```python
from build123d import *

# Parameters (mm, degrees)
F1_DEPTH = 16
F2_R     = 7
F3_T     = -3
F5_DEPTH = 3.1
F6_R     = 0.4


with BuildPart() as f1:
    # F0 (on Top) → F1 (new body)
    with BuildSketch(Plane.XY):
        with BuildLine():
            Line((-44, -34.5), (44, -34.5))
            ThreePointArc((44, -34.5), (48.9497474683, -32.4497474683), (51, -27.5))
            Line((51, -27.5), (51, 27.5))
            ThreePointArc((51, 27.5), (48.9497474683, 32.4497474683), (44, 34.5))
            Line((44, 34.5), (-44, 34.5))
            ThreePointArc((-44, 34.5), (-48.9497474683, 32.4497474683), (-51, 27.5))
            Line((-51, 27.5), (-51, -27.5))
            ThreePointArc((-51, -27.5), (-48.9497474683, -32.4497474683), (-44, -34.5))
        make_face()
    extrude(amount=F1_DEPTH)

    # F2
    f2_edges = [f1.edges().sort_by_distance(p)[0] for p in [
        (0, -34.5, 0),
    ]]
    fillet(f2_edges, radius=F2_R)

    # F3
    f3_openings = [f1.faces().sort_by_distance(p)[0] for p in [
        (0, 0, 16),
    ]]
    offset(amount=F3_T, openings=f3_openings)

    # F4 (on face) → F5 (cut)
    with BuildSketch(Plane.XY.offset(16)):
        with BuildLine():
            Line((49.6, -27.5), (49.6, 27.5))
            ThreePointArc((49.6, 27.5), (47.9597979746, 31.4597979746), (44, 33.1))
            Line((44, 33.1), (-44, 33.1))
            ThreePointArc((-44, 33.1), (-47.9597979746, 31.4597979746), (-49.6, 27.5))
            Line((-49.6, 27.5), (-49.6, -27.5))
            ThreePointArc((-49.6, -27.5), (-47.9597979746, -31.4597979746), (-44, -33.1))
            Line((-44, -33.1), (44, -33.1))
            ThreePointArc((44, -33.1), (47.9597979746, -31.4597979746), (49.6, -27.5))
        make_face()
        with BuildLine():
            Line((-44, 31.5), (44, 31.5))
            ThreePointArc((44, 31.5), (46.8284271247, 30.3284271247), (48, 27.5))
            Line((48, 27.5), (48, -27.5))
            ThreePointArc((48, -27.5), (46.8284271247, -30.3284271247), (44, -31.5))
            Line((44, -31.5), (-44, -31.5))
            ThreePointArc((-44, -31.5), (-46.8284271247, -30.3284271247), (-48, -27.5))
            Line((-48, -27.5), (-48, 27.5))
            ThreePointArc((-48, 27.5), (-46.8284271247, 30.3284271247), (-44, 31.5))
        make_face(mode=Mode.SUBTRACT)
    extrude(amount=-F5_DEPTH, mode=Mode.SUBTRACT)

    # F6
    f6_edges = [f1.edges().sort_by_distance(p)[0] for p in [
        (0, 33.1, 12.9),
        (0, -33.1, 16),
    ]]
    fillet(f6_edges, radius=F6_R)


solid = f1.part
```
Can you work these out from the model? Positions are in its coordinate system, mm. A direction names the side the tool comes from. Give positions to 0.01 mm unless a question says otherwise; leave off trailing zeros. Write each loop counter-clockwise with the first axis right and the second up, starting at its lowest first coordinate (ties: lowest second). Pieces come first, ordered by that corner, then holes. Notation, with made-up numbers: (62, 82.5) -> (107, 82.5) arc R23 ccw to (107, 97.5) -> close; hole circle Ø8 at (-29, 40). An arc over 180 degrees is marked (long way). One line per item, written item: value.
Q1. We'd pull the mould along X, two halves only. Please class faces 3 (the face through (-1, 0, 3)), 4 (the face through (48, 31.42, 14.47)), 5 (the face through (-49, -32.4, 11.4)), 6 (the face through (51, 0, 11)): +X half, -X half, draft (parallel to the pull), parting line (faces both ways), or undercut.
Results found:
face 3: undercut
face 4: undercut
face 5: -X half
face 6: +X half
Q2. Imagine slicing it at A-A on z = 10. Please give me the cut outline in (x, y).
Results found:
outline: (-51, -27.5) arc R7 ccw to (-44, -34.5) -> (44, -34.5) arc R7 ccw to (51, -27.5) -> (51, 27.5) arc R7 ccw to (44, 34.5) -> (-44, 34.5) arc R7 ccw to (-51, 27.5) -> close; hole (-48, -27.5) arc R4 ccw to (-44, -31.5) -> (44, -31.5) arc R4 ccw to (48, -27.5) -> (48, 27.5) arc R4 ccw to (44, 31.5) -> (-44, 31.5) arc R4 ccw to (-48, 27.5) -> close
Q3. Imagine slicing it at B-B on y = 24. Please give me the cut outline in (x, z), and give its area (3 significant figures).
Results found:
outline: (-51, 7) arc R7 ccw to (-44, 0) -> (44, 0) arc R7 ccw to (51, 7) -> (51, 16) -> (50, 16) arc R0.4 ccw to (49.6, 15.6) -> (49.6, 13.3) arc R0.4 cw to (49.2, 12.9) -> (48, 12.9) -> (48, 7) arc R4 cw to (44, 3) -> (-44, 3) arc R4 cw to (-48, 7) -> (-48, 12.9) -> (-49.2, 12.9) arc R0.4 cw to (-49.6, 13.3) -> (-49.6, 15.6) arc R0.4 ccw to (-50, 16) -> (-51, 16) -> close
area: 360 mm^2
Q4. Imagine slicing it at C-C on x = -18.5. Please give me the cut outline in (y, z), and give its area (3 significant figures).
Results found:
outline: (-34.5, 7) arc R7 ccw to (-27.5, 0) -> (27.5, 0) arc R7 ccw to (34.5, 7) -> (34.5, 16) -> (33.5, 16) arc R0.4 ccw to (33.1, 15.6) -> (33.1, 13.3) arc R0.4 cw to (32.7, 12.9) -> (31.5, 12.9) -> (31.5, 7) arc R4 cw to (27.5, 3) -> (-27.5, 3) arc R4 cw to (-31.5, 7) -> (-31.5, 12.9) -> (-32.7, 12.9) arc R0.4 cw to (-33.1, 13.3) -> (-33.1, 15.6) arc R0.4 ccw to (-33.5, 16) -> (-34.5, 16) -> close
area: 261 mm^2
Q5. Please list where these lines run through material, in increasing order: line 1 (Y direction, x = 40.5, z = 15); line 2 (Y direction, x = -20, z = 11.5); line 3 (X direction, y = 20.5, z = 12.5). Write a range as [from, to].
Results found:
line 1: y = [-34.5, -33.1], [33.1, 34.5]
line 2: y = [-34.5, -31.5], [31.5, 34.5]
line 3: x = [-51, -48], [48, 51]
Q6. Which directions (+Z, -Z, +X, -X, +Y, -Y) give clear straight access to the entire face, cutting with the end or side of a thin tool? Please do faces 1 (the face through (3, 32, 12.9)), 2 (the face through (0.6, -32.5, 2.1)).
Results found:
face 1: +Z
face 2: -Z, +X, -X, -Y
Q7. Imagine slicing it at D-D on z = 14.5. Please give me the cut outline in (x, y), and give its area (3 significant figures).
Results found:
outline: (-51, -27.5) arc R7 ccw to (-44, -34.5) -> (44, -34.5) arc R7 ccw to (51, -27.5) -> (51, 27.5) arc R7 ccw to (44, 34.5) -> (-44, 34.5) arc R7 ccw to (-51, 27.5) -> close; hole (-49.6, -27.5) arc R5.6 ccw to (-44, -33.1) -> (44, -33.1) arc R5.6 ccw to (49.6, -27.5) -> (49.6, 27.5) arc R5.6 ccw to (44, 33.1) -> (-44, 33.1) arc R5.6 ccw to (-49.6, 27.5) -> close
area: 456 mm^2
Q8. For P1, Ø3, axis at x = -17.5, y = 12, coming from the +Z side, with a flat end and sliding along its axis, tell me the tip position at first contact or that it passes through.
Results found:
P1: stops at z = 3
